Can you work these out from the model? Positions are in its coordinate system, mm. Face numbers are marked on the shaded views. A direction names the side the tool comes from. Give positions to 0.01 mm unless a question says otherwise; leave off trailing zeros. Write each loop counter-clockwise with the first axis right and the second up, starting at its lowest first coordinate (ties: lowest second). Pieces come first, ordered by that corner, then holes. Notation, with made-up numbers: (-37.75, 77) - (-1.75, 77) arc R12 cw to (-1.75, 94) - close; hole circle Ø6 at (84.5, -27.5). An arc over 180 degrees is marked (long way). Use a Markdown table: item, result. Add a question column.
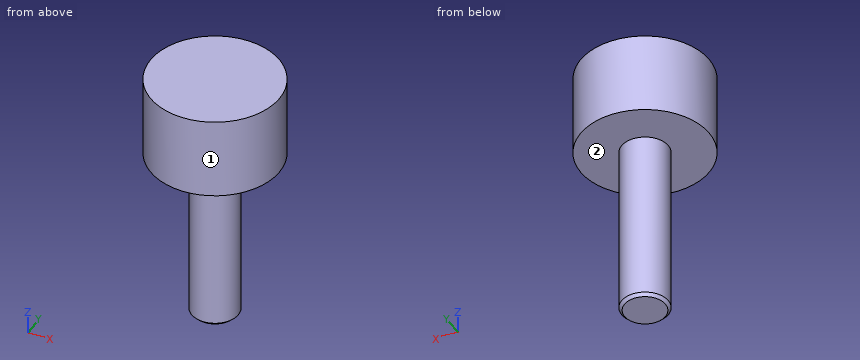
```python
from build123d import *

# Parameters (mm, degrees)
F0_R     = 11
F1_DEPTH = 14
F2_R     = 3.99
F3_DEPTH = 30
F4_SIZE  = 0.5


with BuildPart() as f1:
    # F0 (on Top) → F1 (new body)
    with BuildSketch(Plane.XY):
        Circle(F0_R)
    extrude(amount=F1_DEPTH)

    # F2 (on Top) → F3 (join)
    with BuildSketch(Plane.XY):
        Circle(F2_R)
    extrude(amount=-F3_DEPTH)

    # F4
    f4_edges = [f1.edges().sort_by_distance(p)[0] for p in [
        (-3.99, 0, -30),
    ]]
    chamfer(f4_edges, length=F4_SIZE)


solid = f1.part
```
Q1. Suppose I cut it at A-A (y = 0). Please give me the cut outline in (x, z), and give its area (3 significant figures).
Q2. I'm going to push flat-ended pins straight in: P1, Ø12, axis at x = -1, y = 5, coming from the -Z side; P2, Ø5, axis at y = 6, z = -6, coming from the -X side; P3, Ø3, axis at x = 6, y = 5.5, coming from the -Z side; P4, Ø10, axis at y = 0.5, z = -6.5, coming from the -X side. Where does each tip first touch, or does it pass through?
Q3. On a 3-axis mill with a long thin cutter (end or side, diameter ignored), from which of +Z, -Z, +X, -X, +Y, -Y can I reach the whole of each face in a straight line? I mean the marked faces 1 and 2. Say none if no direction works.
Q4. If I drill on probe 1 along Z at (x, y) = (-1, 9); probe 2 along Y at (x, z) = (1.5, -8); probe 3 along Y at (x, z) = (2.5, -10), over which ranges is the centre line in solid material (lowest first)? Write a range as [from, to].
Q5. Suppose I cut it at D-D (z = -13). Please give me the cut outline in (x, y), and give its area (3 significant figures).
Q6. Suppose I cut it at C-C (z = 1). Please give me the cut outline in (x, y).
Derived:
| question | item | result |
|---|---|---|
| 1 | outline | (-11, 0) - (-3.99, 0) - (-3.99, -29.5) - (-3.49, -30) - (3.49, -30) - (3.99, -29.5) - (3.99, 0) - (11, 0) - (11, 14) - (-11, 14) - close |
| 1 | area | 547 mm² |
| 2 | P1 | z = -30 |
| 2 | P2 | x = -1.92 |
| 2 | P3 | z = 0 |
| 2 | P4 | x = -3.99 |
| 3 | face 1 | +Z, -Z |
| 3 | face 2 | -Z |
| 4 | probe 1 | [0, 14] |
| 4 | probe 2 | [-3.7, 3.7] |
| 4 | probe 3 | [-3.11, 3.11] |
| 5 | outline | circle Ø7.98 at (0, 0) |
| 5 | area | 50.0 mm² |
| 6 | outline | circle Ø22 at (0, 0) |
